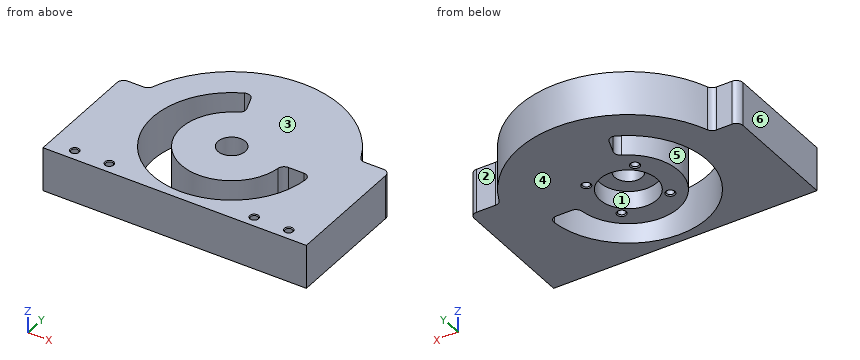
from build123d import *

# Parameters (mm, degrees)
SKIZZE1_R                       = 6.25
AUFSATZ_LINEAR_AUSTRAGEN1_DEPTH = 20
SKIZZE4_R                       = 13
SCHNITT_LINEAR_AUSTRAGEN2_DEPTH = 8
SCHNITT_LINEAR_AUSTRAGEN3_DEPTH = 34.3
VERRUNDUNG1_R                   = 3
VERRUNDUNG2_R                   = 3
SKIZZE7_R                       = 1
SCHNITT_LINEAR_AUSTRAGEN5_DEPTH = 15
M4_GEWINDEBOHRUNG3_D            = 3.3
M4_GEWINDEBOHRUNG3_DEPTH        = 11.5
M4_GEWINDEBOHRUNG3_CSINK_D      = 4.25
M4_GEWINDEBOHRUNG3_CSINK_ANGLE  = 90
M4_GEWINDEBOHRUNG3_TIP          = 0.991420021
M4_GEWINDEBOHRUNG4_D            = 3.3
M4_GEWINDEBOHRUNG4_DEPTH        = 11.5
M4_GEWINDEBOHRUNG4_CSINK_D      = 4.05
M4_GEWINDEBOHRUNG4_CSINK_ANGLE  = 90
M4_GEWINDEBOHRUNG4_TIP          = 0.991420021


with BuildPart() as part:
    # Skizze1 → Aufsatz-Linear austragen1 (new body)
    with BuildSketch(Plane.XY):
        with BuildLine():
            Line((0, 0), (120, 0))
            Line((120, 0), (120, 58.75))
            Line((120, 58.75), (106.351240544, 58.75))
            ThreePointArc((106.351240544, 58.75), (58.007924384, 89.960300587), (12.303039929, 55))
            Line((12.303039929, 55), (0, 55))
            Line((0, 55), (0, 0))
        make_face()
        with Locations((60, 40)):
            Circle(SKIZZE1_R, mode=Mode.SUBTRACT)
    extrude(amount=AUFSATZ_LINEAR_AUSTRAGEN1_DEPTH)

    # Skizze4 → Schnitt-Linear austragen2 (cut)
    with BuildSketch(Plane(origin=(0, 0, 0), x_dir=(-1, 0, 0), z_dir=(0, 0, -1))):
        with Locations((-60, 40)):
            Circle(SKIZZE4_R)
    extrude(amount=-SCHNITT_LINEAR_AUSTRAGEN2_DEPTH, mode=Mode.SUBTRACT)

    # Skizze5 → Schnitt-Linear austragen3 (cut)
    with BuildSketch(Plane(origin=(0, 0, 0), x_dir=(-1, 0, 0), z_dir=(0, 0, -1))):
        with BuildLine():
            Line((-96, 40), (-83, 40))
            ThreePointArc((-83, 40), (-46.807741964, 21.159502981), (-52.133536704, 61.612930278))
            Line((-52.133536704, 61.612930278), (-47.68727484, 73.828934348))
            ThreePointArc((-47.68727484, 73.828934348), (-39.351248291, 10.510526406), (-96, 40))
        make_face()
    extrude(amount=-SCHNITT_LINEAR_AUSTRAGEN3_DEPTH, mode=Mode.SUBTRACT)

    # Verrundung1
    verrundung1_edges = [part.edges().sort_by_distance(p)[0] for p in [
        (47.68727484, 73.828934348, 10),
        (96, 40, 10),
        (83, 40, 10),
        (52.133536704, 61.612930278, 10),
    ]]
    fillet(verrundung1_edges, radius=VERRUNDUNG1_R)

    # Verrundung2
    verrundung2_edges = [part.edges().sort_by_distance(p)[0] for p in [
        (0, 55, 10),
        (12.303039929, 55, 10),
        (106.351240544, 58.75, 10),
        (120, 58.75, 10),
    ]]
    fillet(verrundung2_edges, radius=VERRUNDUNG2_R)

    # Skizze7 → Schnitt-Linear austragen5 (cut)
    with BuildSketch(Plane(origin=(0, 0, 0), x_dir=(-1, 0, 0), z_dir=(0, 0, -1))):
        with Locations((-72.0838337, 50.8848961)):
            Circle(SKIZZE7_R)
        with Locations((-49.1151039, 52.0838337)):
            Circle(SKIZZE7_R)
        with Locations((-70.8848961, 27.9161663)):
            Circle(SKIZZE7_R)
        with Locations((-47.9161663, 29.1151039)):
            Circle(SKIZZE7_R)
    extrude(amount=-SCHNITT_LINEAR_AUSTRAGEN5_DEPTH, mode=Mode.SUBTRACT)

    # M4 Gewindebohrung3
    with Locations(Plane(origin=(72.0838337, 50.8848961, 0), x_dir=(-1, 0, 0), z_dir=(0, 0, -1))):
        with Locations((0, 0), (22.9687298, 1.1989376), (24.1676674, -21.7697922), (1.1989376, -22.9687298)):
            CounterSinkHole(M4_GEWINDEBOHRUNG3_D / 2, M4_GEWINDEBOHRUNG3_CSINK_D / 2, depth=M4_GEWINDEBOHRUNG3_DEPTH, counter_sink_angle=M4_GEWINDEBOHRUNG3_CSINK_ANGLE)
            with Locations((0, 0, -(M4_GEWINDEBOHRUNG3_DEPTH + M4_GEWINDEBOHRUNG3_TIP / 2))):  # 118° drill point
                Cone(0, M4_GEWINDEBOHRUNG3_D / 2, M4_GEWINDEBOHRUNG3_TIP, mode=Mode.SUBTRACT)

    # M4 Gewindebohrung4
    with Locations(Plane(origin=(11.25, 5, 20), x_dir=(1, 0, 0), z_dir=(0, 0, 1))):
        with Locations((0, 0), (15.75, 0), (81.75, 0), (97.5, 0)):
            CounterSinkHole(M4_GEWINDEBOHRUNG4_D / 2, M4_GEWINDEBOHRUNG4_CSINK_D / 2, depth=M4_GEWINDEBOHRUNG4_DEPTH, counter_sink_angle=M4_GEWINDEBOHRUNG4_CSINK_ANGLE)
            with Locations((0, 0, -(M4_GEWINDEBOHRUNG4_DEPTH + M4_GEWINDEBOHRUNG4_TIP / 2))):  # 118° drill point
                Cone(0, M4_GEWINDEBOHRUNG4_D / 2, M4_GEWINDEBOHRUNG4_TIP, mode=Mode.SUBTRACT)


solid = part.part
Check sheet for the modelled part. Datum: model origin and axes. Units: mm. Face numbers are marked on the shaded views. A direction names the side the tool comes from. Coordinates: 2 decimals unless noted, no trailing zeros. Loops run counter-clockwise (first coordinate to the right, second up) from the corner with the lowest first, then second, coordinate; pieces in that order, holes last. Notation, with made-up numbers: (58.5, 86) -> (77.5, 86) arc R28 ccw to (77.5, 119) -> close; hole circle Ø5 at (-34.5, 22.25). An arc over 180 degrees is marked (long way). Answer in a Markdown table with one row per item.
1. Sectioned sample at D-D, the plane x = 33.5. Record the boundary of the cut face in (y, z).
Check values:
| item | result |
|---|---|
| outline | (0, 0) -> (15.63, 0) -> (15.63, 20) -> (0, 20) -> close; (64.37, 0) -> (82.4, 0) -> (82.4, 20) -> (64.37, 20) -> close |
2. Sectioned sample at B-B, the plane y = 10.5. Record the boundary of the cut face in (x, z), then the cut area to 3 significant figures.
Check values:
| item | result |
|---|---|
| outline | (0, 0) -> (39.37, 0) -> (39.37, 20) -> (0, 20) -> close; (80.63, 0) -> (120, 0) -> (120, 20) -> (80.63, 20) -> close |
| area | 1,570 mm2 |
3. Material ranges on line 1 along Y through (x, z) = (60, 5.5); line 2 along Y through (x, z) = (60, 15.5); line 3 along X through (y, z) = (28.5, 13.75), recorded low to high. Write a range as [from, to].
Check values:
| item | result |
|---|---|
| line 1 | y = [0, 4], [17, 27], [53, 90] |
| line 2 | y = [0, 4], [17, 33.75], [46.25, 90] |
| line 3 | x = [0, 25.89], [40.08, 47.13], [48.7, 70.07], [71.7, 79.92], [94.11, 120] |
4. Sectioned sample at A-A, the plane x = 60. Record the boundary of the cut face in (y, z), then the cut area to 3 significant figures.
Check values:
| item | result |
|---|---|
| outline | (0, 0) -> (4, 0) -> (4, 20) -> (0, 20) -> close; (17, 0) -> (27, 0) -> (27, 8) -> (33.75, 8) -> (33.75, 20) -> (17, 20) -> close; (46.25, 8) -> (53, 8) -> (53, 0) -> (90, 0) -> (90, 20) -> (46.25, 20) -> close |
| area | 1,180 mm2 |
5. Go/stop test with flat-tipped pins: pin 1 (23.5 mm diameter, centred on x = 60, y = 40, fed in from -Z); pin 2 (5 mm diameter, centred on y = 67, z = 14, fed in from -X); pin 3 (1 mm diameter, centred on x = 72, y = 50.5, fed in from -Z); pin 4 (11 mm diameter, centred on x = 60, y = 40, fed in from -Z). Record where each tip stops, or that it passes through.
Check values:
| item | result |
|---|---|
| pin 1 | stops at z = 8 |
| pin 2 | stops at x = 16.41 |
| pin 3 | stops at z = 15 |
| pin 4 | passes through |
6. Release check for a two-part mould opening along X. For the marked faces 4, 5 and 6 record: released by +X, released by -X, zero draft, split by the parting line, or undercut.
Check values:
| item | result |
|---|---|
| face 4 | zero draft |
| face 5 | undercut |
| face 6 | released by -X |
7. Access from +Z, -Z, +X, -X, +Y, -Y to the whole of each face (thin tool, end or side, straight path). Record for the marked faces 1, 2 and 3.
Check values:
| item | result |
|---|---|
| face 1 | -Z |
| face 2 | +Z, -Z, +X, +Y |
| face 3 | +Z, +X, -X, +Y, -Y |
8. Sectioned sample at C-C, the plane z = 13.25. Give the number of separate pieces and of enclosed holes in the cut face, then the cut area to 3 significant figures.
Check values:
| item | result |
|---|---|
| separate pieces | 1 |
| enclosed holes | 10 |
| area | 7,260 mm2 |
